Read the model definition and answer for the solid it produces. Units are mm, in the model's axes. Face numbers are marked on the shaded views. A direction names the side the tool comes from. Coordinates: 2 decimals unless noted, no trailing zeros. Order: outer loops, then holes, each group sorted by start corner. A loop starts at its lowest first (then second) coordinate and runs counter-clockwise, first axis right, second up.
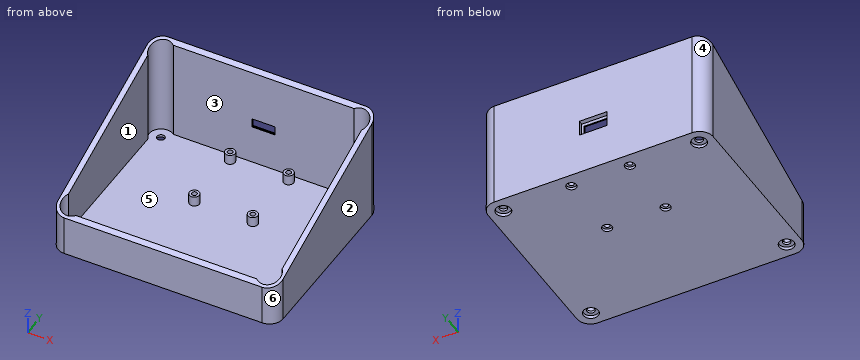
```python
from build123d import *

# Parameters (mm, degrees)
OUTER_R6_DEPTH                         = 55
CAVITY_FLOOR2P5_WALL2P5_START          = 2.5
CAVITY_FLOOR2P5_WALL2P5_DEPTH          = 65
PANEL_SEAT_20DEG_DEPTH                 = 142.707445111
PANEL_SEAT_20DEG_DEPTH_BACK            = 142.707445111
INTERNAL_POST_CLEARANCE_0_START        = 2.5
SKETCH_4_R                             = 5.2
INTERNAL_POST_CLEARANCE_0_DEPTH        = 60
SKETCH_5_R                             = 1.7
UNDERSIDE_M3_0_DEPTH                   = 3
SKETCH_6_R                             = 3.3
UNDERSIDE_HEAD_RECESS_0_DEPTH          = 1.4
INTERNAL_POST_CLEARANCE_1_START        = 2.5
SKETCH_7_R                             = 5.2
INTERNAL_POST_CLEARANCE_1_DEPTH        = 60
SKETCH_8_R                             = 1.7
UNDERSIDE_M3_1_DEPTH                   = 3
SKETCH_9_R                             = 3.3
UNDERSIDE_HEAD_RECESS_1_DEPTH          = 1.4
INTERNAL_POST_CLEARANCE_2_START        = 2.5
SKETCH_10_R                            = 5.2
INTERNAL_POST_CLEARANCE_2_DEPTH        = 60
SKETCH_11_R                            = 1.7
UNDERSIDE_M3_2_DEPTH                   = 3
SKETCH_12_R                            = 3.3
UNDERSIDE_HEAD_RECESS_2_DEPTH          = 1.4
INTERNAL_POST_CLEARANCE_3_START        = 2.5
SKETCH_13_R                            = 5.2
INTERNAL_POST_CLEARANCE_3_DEPTH        = 60
SKETCH_14_R                            = 1.7
UNDERSIDE_M3_3_DEPTH                   = 3
SKETCH_15_R                            = 3.3
UNDERSIDE_HEAD_RECESS_3_DEPTH          = 1.4
CENTERED_CARRIER_SUPPORTS_Z7_START     = 2.5
SKETCH_16_R                            = 2.2
CENTERED_CARRIER_SUPPORTS_Z7_DEPTH     = 4.5
SKETCH_17_R                            = 1.15
CARRIER_M2_CLEARANCE_DEPTH             = 8
SKETCH_18_R                            = 2.2
CARRIER_HEAD_RECESS_DEPTH              = 1.2
USB_C_CENTERED_INNER_OPENING_START     = 80
SKETCH_19_W                            = 10.2
SKETCH_19_H                            = 4.08
USB_C_CENTERED_INNER_OPENING_DEPTH     = 6
USB_PLUG_SHOULDER_SHALLOW_RECESS_START = 82
SKETCH_20_W                            = 12.4
SKETCH_20_H                            = 7
USB_PLUG_SHOULDER_SHALLOW_RECESS_DEPTH = 3


with BuildPart() as part:
    # 草图1 → Outer_R6 (new body)
    with BuildSketch(Plane.XY):
        with BuildLine():
            Line((6, 0), (94, 0))
            ThreePointArc((94, 0), (98.242640687, 1.757359313), (100, 6))
            Line((100, 6), (100, 78))
            ThreePointArc((100, 78), (98.242640687, 82.242640687), (94, 84))
            Line((94, 84), (6, 84))
            ThreePointArc((6, 84), (1.757359313, 82.242640687), (0, 78))
            Line((0, 78), (0, 6))
            ThreePointArc((0, 6), (1.757359313, 1.757359313), (6, 0))
        make_face()
    extrude(amount=OUTER_R6_DEPTH)

    # 草图2 → Cavity_floor2p5_wall2p5 (cut)
    with BuildSketch(Plane.XY.offset(CAVITY_FLOOR2P5_WALL2P5_START)):
        with BuildLine():
            Line((6, 2.5), (94, 2.5))
            ThreePointArc((94, 2.5), (96.474873734, 3.525126266), (97.5, 6))
            Line((97.5, 6), (97.5, 78))
            ThreePointArc((97.5, 78), (96.474873734, 80.474873734), (94, 81.5))
            Line((94, 81.5), (6, 81.5))
            ThreePointArc((6, 81.5), (3.525126266, 80.474873734), (2.5, 78))
            Line((2.5, 78), (2.5, 6))
            ThreePointArc((2.5, 6), (3.525126266, 3.525126266), (6, 2.5))
        make_face()
    extrude(amount=CAVITY_FLOOR2P5_WALL2P5_DEPTH, mode=Mode.SUBTRACT)

    # 草图3 → Panel_seat_20deg (cut, two sides: drawn at the far end of the back side and taken through both)
    with BuildSketch(Plane(origin=(0, 0, 0), x_dir=(0, 0, -1), z_dir=(1, 0, 0)).offset(-PANEL_SEAT_20DEG_DEPTH_BACK)):
        Polygon((-10.720595315, -20), (-58.036725769, 110), (-120, 110), (-120, -20), align=None)
    extrude(amount=PANEL_SEAT_20DEG_DEPTH + PANEL_SEAT_20DEG_DEPTH_BACK, mode=Mode.SUBTRACT)

    # 草图4 → Internal_post_clearance_0 (cut)
    with BuildSketch(Plane.XY.offset(INTERNAL_POST_CLEARANCE_0_START)):
        with Locations((6.5, 6.5)):
            Circle(SKETCH_4_R)
    extrude(amount=INTERNAL_POST_CLEARANCE_0_DEPTH, mode=Mode.SUBTRACT)

    # 草图5 → Underside_M3_0 (cut)
    with BuildSketch(Plane.XY):
        with Locations((6.5, 6.5)):
            Circle(SKETCH_5_R)
    extrude(amount=UNDERSIDE_M3_0_DEPTH, mode=Mode.SUBTRACT)

    # 草图6 → Underside_head_recess_0 (cut)
    with BuildSketch(Plane.XY):
        with Locations((6.5, 6.5)):
            Circle(SKETCH_6_R)
    extrude(amount=UNDERSIDE_HEAD_RECESS_0_DEPTH, mode=Mode.SUBTRACT)

    # 草图7 → Internal_post_clearance_1 (cut)
    with BuildSketch(Plane.XY.offset(INTERNAL_POST_CLEARANCE_1_START)):
        with Locations((93.5, 6.5)):
            Circle(SKETCH_7_R)
    extrude(amount=INTERNAL_POST_CLEARANCE_1_DEPTH, mode=Mode.SUBTRACT)

    # 草图8 → Underside_M3_1 (cut)
    with BuildSketch(Plane.XY):
        with Locations((93.5, 6.5)):
            Circle(SKETCH_8_R)
    extrude(amount=UNDERSIDE_M3_1_DEPTH, mode=Mode.SUBTRACT)

    # 草图9 → Underside_head_recess_1 (cut)
    with BuildSketch(Plane.XY):
        with Locations((93.5, 6.5)):
            Circle(SKETCH_9_R)
    extrude(amount=UNDERSIDE_HEAD_RECESS_1_DEPTH, mode=Mode.SUBTRACT)

    # 草图10 → Internal_post_clearance_2 (cut)
    with BuildSketch(Plane.XY.offset(INTERNAL_POST_CLEARANCE_2_START)):
        with Locations((6.5, 77.5)):
            Circle(SKETCH_10_R)
    extrude(amount=INTERNAL_POST_CLEARANCE_2_DEPTH, mode=Mode.SUBTRACT)

    # 草图11 → Underside_M3_2 (cut)
    with BuildSketch(Plane.XY):
        with Locations((6.5, 77.5)):
            Circle(SKETCH_11_R)
    extrude(amount=UNDERSIDE_M3_2_DEPTH, mode=Mode.SUBTRACT)

    # 草图12 → Underside_head_recess_2 (cut)
    with BuildSketch(Plane.XY):
        with Locations((6.5, 77.5)):
            Circle(SKETCH_12_R)
    extrude(amount=UNDERSIDE_HEAD_RECESS_2_DEPTH, mode=Mode.SUBTRACT)

    # 草图13 → Internal_post_clearance_3 (cut)
    with BuildSketch(Plane.XY.offset(INTERNAL_POST_CLEARANCE_3_START)):
        with Locations((93.5, 77.5)):
            Circle(SKETCH_13_R)
    extrude(amount=INTERNAL_POST_CLEARANCE_3_DEPTH, mode=Mode.SUBTRACT)

    # 草图14 → Underside_M3_3 (cut)
    with BuildSketch(Plane.XY):
        with Locations((93.5, 77.5)):
            Circle(SKETCH_14_R)
    extrude(amount=UNDERSIDE_M3_3_DEPTH, mode=Mode.SUBTRACT)

    # 草图15 → Underside_head_recess_3 (cut)
    with BuildSketch(Plane.XY):
        with Locations((93.5, 77.5)):
            Circle(SKETCH_15_R)
    extrude(amount=UNDERSIDE_HEAD_RECESS_3_DEPTH, mode=Mode.SUBTRACT)

    # 草图16 → Centered_carrier_supports_Z7 (add)
    with BuildSketch(Plane.XY.offset(CENTERED_CARRIER_SUPPORTS_Z7_START)):
        with Locations((37, 49)):
            Circle(SKETCH_16_R)
        with Locations((63, 49)):
            Circle(SKETCH_16_R)
        with Locations((37, 78)):
            Circle(SKETCH_16_R)
        with Locations((63, 78)):
            Circle(SKETCH_16_R)
    extrude(amount=CENTERED_CARRIER_SUPPORTS_Z7_DEPTH)

    # 草图17 → Carrier_M2_clearance (cut)
    with BuildSketch(Plane.XY):
        with Locations((37, 49)):
            Circle(SKETCH_17_R)
        with Locations((63, 49)):
            Circle(SKETCH_17_R)
        with Locations((37, 78)):
            Circle(SKETCH_17_R)
        with Locations((63, 78)):
            Circle(SKETCH_17_R)
    extrude(amount=CARRIER_M2_CLEARANCE_DEPTH, mode=Mode.SUBTRACT)

    # 草图18 → Carrier_head_recess (cut)
    with BuildSketch(Plane.XY):
        with Locations((37, 49)):
            Circle(SKETCH_18_R)
        with Locations((63, 49)):
            Circle(SKETCH_18_R)
        with Locations((37, 78)):
            Circle(SKETCH_18_R)
        with Locations((63, 78)):
            Circle(SKETCH_18_R)
    extrude(amount=CARRIER_HEAD_RECESS_DEPTH, mode=Mode.SUBTRACT)

    # 草图19 → USB_C_centered_inner_opening (cut)
    with BuildSketch(Plane(origin=(0, 0, 0), x_dir=(1, 0, 0), z_dir=(0, 1, 0)).offset(USB_C_CENTERED_INNER_OPENING_START)):
        with Locations((50, -22.29)):
            Rectangle(SKETCH_19_W, SKETCH_19_H)
    extrude(amount=USB_C_CENTERED_INNER_OPENING_DEPTH, mode=Mode.SUBTRACT)

    # 草图20 → USB_plug_shoulder_shallow_recess (cut)
    with BuildSketch(Plane(origin=(0, 0, 0), x_dir=(1, 0, 0), z_dir=(0, 1, 0)).offset(USB_PLUG_SHOULDER_SHALLOW_RECESS_START)):
        with Locations((50, -22.29)):
            Rectangle(SKETCH_20_W, SKETCH_20_H)
    extrude(amount=USB_PLUG_SHOULDER_SHALLOW_RECESS_DEPTH, mode=Mode.SUBTRACT)


solid = part.part
```
1) Straight lines are drawn through the part: line 1 (Y direction, x = 93.5, z = 1.7); line 2 (Y direction, x = 63, z = 0.55); line 3 (X direction, y = 34, z = 14.5). For each, find the intervals that lie inside material, in ascending order.
A:
line 1: y = 0 to 4.8, 8.2 to 75.8, 79.2 to 84
line 2: y = 0 to 46.8, 51.2 to 75.8, 80.2 to 84
line 3: x = 0 to 2.5, 97.5 to 100
2) Which of the six approach directions +Z, -Z, +X, -X, +Y, -Y give full straight-line access (tool end or side, diameter ignored) to the marked faces 1 and 2?
A:
face 1: +Z
face 2: +Z, -Z, +X, +Y, -Y
3) A cutting plane is placed at A-A, the plane x = 63. State how many separate pieces and enclosed holes the cut face has, and give its area (3 significant figures).
A:
separate pieces: 3
enclosed holes: 0
area: 366 mm2
4) Flat-ended cylindrical pins translate along their axes: pin 1 Ø2 at (x, y) = (37, 78.5) entering from -Z; pin 2 Ø2 at (x, y) = (51.5, 82.5) entering from -Z; pin 3 Ø5 at (x, y) = (88.5, 21.5) entering from +Z; pin 4 Ø4 at (x, y) = (6.5, 77.5) entering from -Z. Find the tip coordinate at first contact, or state that the pin passes through.
A:
pin 1: stops at z = 1.2
pin 2: stops at z = 0
pin 3: stops at z = 2.5
pin 4: stops at z = 1.4
5) A cutting plane is placed at B-B, the plane z = 14. Determine the outline of the cut face in (x, y), and give its area (3 significant figures).
A:
outline: (0, 6) arc R6 ccw to (6, 0) - (94, 0) arc R6 ccw to (100, 6) - (100, 78) arc R6 ccw to (94, 84) - (6, 84) arc R6 ccw to (0, 78) - close; hole (2.5, 9.82) arc R5.2 ccw to (9.82, 2.5) - (90.18, 2.5) arc R5.2 ccw to (97.5, 9.82) - (97.5, 74.18) arc R5.2 ccw to (90.18, 81.5) - (9.82, 81.5) arc R5.2 ccw to (2.5, 74.18) - close
area: 821 mm2
6) Determine the mould class of the marked faces 3, 4, 5 and 6 for opening direction Y: pulls with the +Y half, pulls with the -Y half, needs draft (parallel to the pull), parting line crosses it, or undercut.
A:
face 3: undercut
face 4: pulls with the +Y half
face 5: undercut
face 6: pulls with the -Y half
7) A cutting plane is placed at C-C, the plane z = 23. Determine the outline of the cut face in (x, y), and give its area (3 significant figures).
A:
outline: (0, 13.74) - (2.5, 13.74) - (2.5, 74.18) arc R5.2 cw to (9.82, 81.5) - (44.9, 81.5) - (44.9, 82) - (43.8, 82) - (43.8, 84) - (6, 84) arc R6 ccw to (0, 78) - close; (55.1, 81.5) - (90.18, 81.5) arc R5.2 cw to (97.5, 74.18) - (97.5, 13.74) - (100, 13.74) - (100, 78) arc R6 ccw to (94, 84) - (56.2, 84) - (56.2, 82) - (55.1, 82) - close
area: 522 mm2
8) A cutting plane is placed at D-D, the plane y = 36. Determine the outline of the cut face in (x, z).
A:
outline: (0, 0) - (100, 0) - (100, 31.1) - (97.5, 31.1) - (97.5, 2.5) - (2.5, 2.5) - (2.5, 31.1) - (0, 31.1) - close
